Geometry check sheet. Reference: the model listing, model coordinates, mm. A direction names the side the tool comes from. Coordinates: 2 decimals unless noted, no trailing zeros. Loops run counter-clockwise (first coordinate to the right, second up) from the corner with the lowest first, then second, coordinate; pieces in that order, holes last. Notation, with made-up numbers: (84.25, 72.25) - (100.25, 72.25) arc R21 cw to (100.25, 111.25) - close; hole circle Ø6 at (-30, 59). An arc over 180 degrees is marked (long way). Write item = value, one per line. Start each with the question number.
from build123d import *

# Parameters (mm, degrees)
F1_DEPTH = 2
F2_R     = 5
F4_DEPTH = 2
F6_DEPTH = 25


# Not quite as in the source:
# - a feature names something its author has since deleted; it is built from what else it names


with BuildPart() as f1:
    # F0 (on Front) → F1 (new body)
    with BuildSketch(Plane.XZ):
        with BuildLine():
            Line((0, 5.5), (0, 0))
            Line((0, 0), (40, 0))
            Line((40, 0), (40, 5.5))
            Line((40, 5.5), (25, 5.5))
            ThreePointArc((25, 5.5), (22, 2.5), (19, 5.5))
            Line((19, 5.5), (0, 5.5))
        make_face()
        with BuildLine():
            Line((40, 5.5), (40, 0))
            Line((40, 0), (40, -2.5))
            ThreePointArc((40, -2.5), (41.05572809, 1.972135955), (44, 5.5))
            Line((44, 5.5), (40, 5.5))
        make_face()
        with BuildLine():
            Line((0, 11), (0, 5.5))
            Line((0, 5.5), (19, 5.5))
            ThreePointArc((19, 5.5), (22, 8.5), (25, 5.5))
            Line((25, 5.5), (40, 5.5))
            Line((40, 5.5), (40, 11))
            Line((40, 11), (0, 11))
        make_face()
        with BuildLine():
            Line((40, 11), (40, 5.5))
            Line((40, 5.5), (44, 5.5))
            ThreePointArc((44, 5.5), (41.05572809, 9.027864045), (40, 13.5))
            Line((40, 13.5), (40, 11))
        make_face()
        with BuildLine():
            Line((45, -2.5), (40, -2.5))
            ThreePointArc((40, -2.5), (50, -12.5), (60, -2.5))
            ThreePointArc((60, -2.5), (58.94427191, 1.972135955), (56, 5.5))
            ThreePointArc((56, 5.5), (53.1622776602, 4.0131670195), (50, 3.5))
            Line((50, 3.5), (50, 2.5))
            ThreePointArc((50, 2.5), (53.5355339059, 1.0355339059), (55, -2.5))
            ThreePointArc((55, -2.5), (50, -7.5), (45, -2.5))
        make_face()
        with BuildLine():
            ThreePointArc((44, 5.5), (41.05572809, 1.972135955), (40, -2.5))
            Line((40, -2.5), (45, -2.5))
            ThreePointArc((45, -2.5), (46.4644660941, 1.0355339059), (50, 2.5))
            Line((50, 2.5), (50, 3.5))
            ThreePointArc((50, 3.5), (46.8377223398, 4.0131670195), (44, 5.5))
        make_face()
        with BuildLine():
            ThreePointArc((40, 13.5), (41.05572809, 9.027864045), (44, 5.5))
            ThreePointArc((44, 5.5), (46.8377223398, 6.9868329805), (50, 7.5))
            Line((50, 7.5), (50, 8.5))
            ThreePointArc((50, 8.5), (46.4644660941, 9.9644660941), (45, 13.5))
            Line((45, 13.5), (40, 13.5))
        make_face()
        with BuildLine():
            Line((50, 5.5), (44, 5.5))
            ThreePointArc((44, 5.5), (46.8377223398, 4.0131670195), (50, 3.5))
            Line((50, 3.5), (50, 5.5))
        make_face()
        with BuildLine():
            ThreePointArc((50, 7.5), (46.8377223398, 6.9868329805), (44, 5.5))
            Line((44, 5.5), (50, 5.5))
            Line((50, 5.5), (50, 7.5))
        make_face()
        with BuildLine():
            ThreePointArc((60, 13.5), (50, 23.5), (40, 13.5))
            Line((40, 13.5), (45, 13.5))
            ThreePointArc((45, 13.5), (50, 18.5), (55, 13.5))
            ThreePointArc((55, 13.5), (53.5355339059, 9.9644660941), (50, 8.5))
            Line((50, 8.5), (50, 7.5))
            ThreePointArc((50, 7.5), (53.1622776602, 6.9868329805), (56, 5.5))
            ThreePointArc((56, 5.5), (58.94427191, 9.027864045), (60, 13.5))
        make_face()
        with BuildLine():
            ThreePointArc((56, 5.5), (53.1622776602, 6.9868329805), (50, 7.5))
            Line((50, 7.5), (50, 5.5))
            Line((50, 5.5), (56, 5.5))
        make_face()
        with BuildLine():
            Line((50, 5.5), (50, 3.5))
            ThreePointArc((50, 3.5), (53.1622776602, 4.0131670195), (56, 5.5))
            Line((56, 5.5), (50, 5.5))
        make_face()
    extrude(amount=F1_DEPTH)

    # F2
    f2_edges = [f1.edges().sort_by_distance(p)[0] for p in [
        (40, -1, 11),
        (0, -1, 11),
        (0, -1, 0),
    ]]
    fillet(f2_edges, radius=F2_R)

    # F3 (on face) → F4 (cut, through all)
    with BuildSketch(Plane.XZ.offset(2)):
        with BuildLine():
            Line((19.0419601085, 6), (0, 6))
            Line((0, 6), (0, 5))
            Line((0, 5), (19.0419601085, 5))
            ThreePointArc((19.0419601085, 5), (19, 5.5), (19.0419601085, 6))
        make_face()
        with BuildLine():
            Line((30, 6), (24.9580398915, 6))
            ThreePointArc((24.9580398915, 6), (24.9894915684, 5.7508787808), (25, 5.5))
            ThreePointArc((25, 5.5), (24.9894915684, 5.2491212192), (24.9580398915, 5))
            Line((24.9580398915, 5), (30, 5))
            Line((30, 5), (30, 6))
        make_face()
    extrude(amount=-F4_DEPTH, mode=Mode.SUBTRACT)

    # F5 (on face) → F6 (cut)
    with BuildSketch(Plane.XZ.offset(2)):
        with BuildLine():
            ThreePointArc((40, -2.5), (40.2109368707, -4.5430964369), (40.8348486101, -6.5))
            Line((40.8348486101, -6.5), (42.3348486101, -6.5))
            Line((42.3348486101, -6.5), (42.3348486101, 0))
            Line((42.3348486101, 0), (40.3175416345, 0))
            ThreePointArc((40.3175416345, 0), (40.0797030373, -1.2399570752), (40, -2.5))
        make_face()
        with BuildLine():
            ThreePointArc((40, -2.5), (40.0797030373, -1.2399570752), (40.3175416345, 0))
            Line((40.3175416345, 0), (40, 0))
            Line((40, 0), (40, -2.5))
        make_face()
    extrude(amount=-F6_DEPTH, mode=Mode.SUBTRACT)


solid = f1.part
(1) Depth check by flat-ended pin: pin 1 (0.5 mm diameter, centred on y = -1.5, z = 5.5, fed in from -X); pin 2 (1 mm diameter, centred on y = -2, z = -6, fed in from +X); pin 3 (1 mm diameter, centred on x = 28.5, y = -1, fed in from -Z). Enter the tip coordinate at first touch or a pass-through.
(2) Sectioned sample at B-B on z = 1.5. Enter the section's corners in (x, y), plus the area to 3 significant figures.
(3) Draft check along Z on faces 4 (the face through (1, -1, 2)), 5 (the face through (20, -1, 11)), 6 (the face through (36, 0, 6)), 7 (the face through (27, -1, 5)). Enter one of: pulls with the +Z half, pulls with the -Z half, needs draft (parallel to the pull), parting line crosses it, or undercut.
(4) Scan lines: line 1 (Z direction, x = 25.5, y = -1.7); line 2 (X direction, y = -0.4, z = -3.5); line 3 (Z direction, x = 46.5, y = -1.05). Record each from-to range of solid material in increasing order.
(5) Tool access check on faces 1 (the face through (2, -1, 10)), 2 (the face through (22.1, -1, 2.5)), 3 (the face through (42.335, -1, -3)). Record the directions out of +Z, -Z, +X, -X, +Y, -Y that give a thin tool (end or side, any length) a straight path to the whole face; none if there is none.
(6) Sectioned sample at C-C on y = -1.5. Count the separate pieces of the cut face and the enclosed holes in it, plus the area to 3 significant figures.
(7) Sectioned sample at A-A on x = 13. Enter the section's corners in (y, z), plus the area to 3 significant figures.
Working result:
q1.pin_1 = 30
q1.pin_2 = 59.54
q1.pin_3 = 0
q2.outline = (1.43, -2) - (47, -2) - (47, 0) - (1.43, 0) - close; (53, -2) - (59.17, -2) - (59.17, 0) - (53, 0) - close
q2.area = 103 mm2
q3.face_4 = pulls with the -Z half
q3.face_5 = pulls with the +Z half
q3.face_6 = needs draft
q3.face_7 = undercut
q4.line_1 = 0 to 5, 6 to 11
q4.line_2 = 42.33 to 45.1, 54.9 to 59.95
q4.line_3 = -11.87 to -6.07, 1.07 to 9.93, 17.07 to 22.87
q5.face_1 = +Z, -X, +Y, -Y
q5.face_2 = +Y, -Y
q5.face_3 = -X, +Y, -Y
q6.separate_pieces = 1
q6.enclosed_holes = 2
q6.area = 825 mm2
q7.outline = (-2, 0) - (0, 0) - (0, 5) - (-2, 5) - close; (-2, 6) - (0, 6) - (0, 11) - (-2, 11) - close
q7.area = 20.0 mm2
